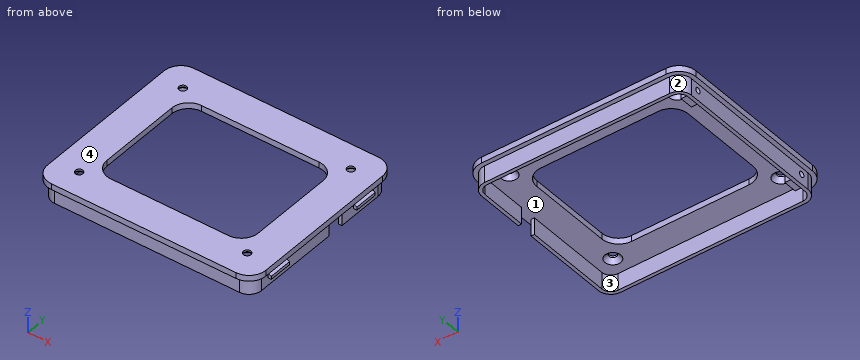
from build123d import *

# Parameters (mm, degrees)
P_IDAT_VYSUNUT_M2_DEPTH                           = 3.5
P_IDAT_VYSUNUT_M3_DEPTH                           = 10
V_LCOV_ZAHLOUBEN_PRO_M4_ROUBY_S_P_2_COUNT         = 2
V_LCOV_ZAHLOUBEN_PRO_M4_ROUBY_S_P_2_PITCH         = 100
V_LCOV_ZAHLOUBEN_PRO_M4_ROUBY_S_P_3_COUNT         = 2
V_LCOV_ZAHLOUBEN_PRO_M4_ROUBY_S_P_3_PITCH         = 128.062484749
V_LCOV_ZAHLOUBEN_PRO_M4_ROUBY_S_P_4_COUNT         = 2
V_LCOV_ZAHLOUBEN_PRO_M4_ROUBY_S_P_4_PITCH         = 80
ODEBRAT_VYSUNUT_M2_DEPTH                          = 86.732140997
SKICA8_W                                          = 5
SKICA8_H                                          = 8
SKICA8_W_2                                        = 3
SKICA8_W_3                                        = 8
P_IDAT_VYSUNUT_M4_DEPTH                           = 5
V_LCOV_ZAHLOUBEN_PRO_M3_ROUBY_S_V_LCO_D           = 3.4
V_LCOV_ZAHLOUBEN_PRO_M3_ROUBY_S_V_LCO_DEPTH       = 9.6
V_LCOV_ZAHLOUBEN_PRO_M3_ROUBY_S_V_LCO_CBORE_D     = 3.9
V_LCOV_ZAHLOUBEN_PRO_M3_ROUBY_S_V_LCO_CBORE_DEPTH = 4
SKICA15_W                                         = 2.8
SKICA15_H                                         = 14
P_IDAT_VYSUNUT_M5_DEPTH                           = 2
ZKOSEN_1_SIZE                                     = 2.144506921
ZKOSEN_1_SIZE_2                                   = 1
ZKOSEN_2_SIZE                                     = 1
ZKOSEN_2_SIZE_2                                   = 2.144506921


with BuildPart() as part:
    # Skica1 → Přidat vysunutím2 (new body)
    with BuildSketch(Plane.XY):
        with BuildLine():
            Line((-55, 55), (55, 55))
            ThreePointArc((55, 55), (62.071067812, 52.071067812), (65, 45))
            Line((65, 45), (65, -45))
            ThreePointArc((65, -45), (62.071067812, -52.071067812), (55, -55))
            Line((55, -55), (-55, -55))
            ThreePointArc((-55, -55), (-62.071067812, -52.071067812), (-65, -45))
            Line((-65, -45), (-65, 45))
            ThreePointArc((-65, 45), (-62.071067812, 52.071067812), (-55, 55))
        make_face()
    extrude(amount=P_IDAT_VYSUNUT_M2_DEPTH)

    # Skica3 → Přidat vysunutím3 (add)
    with BuildSketch(Plane(origin=(0, 0, 0), x_dir=(-1, 0, 0), z_dir=(0, 0, -1))):
        with BuildLine():
            Line((-60.4, 17), (-60.4, 45))
            ThreePointArc((-60.4, 45), (-58.818376618, 48.818376618), (-55, 50.4))
            Line((-55, 50.4), (55, 50.4))
            ThreePointArc((55, 50.4), (58.818376618, 48.818376618), (60.4, 45))
            Line((60.4, 45), (60.4, -45))
            ThreePointArc((60.4, -45), (58.818376618, -48.818376618), (55, -50.4))
            Line((55, -50.4), (-55, -50.4))
            ThreePointArc((-55, -50.4), (-58.818376618, -48.818376618), (-60.4, -45))
            Line((-60.4, -45), (-60.4, 7))
            Line((-60.4, 7), (-62.4, 7))
            Line((-62.4, 7), (-62.4, -45))
            ThreePointArc((-62.4, -45), (-60.232590181, -50.232590181), (-55, -52.4))
            Line((-55, -52.4), (55, -52.4))
            ThreePointArc((55, -52.4), (60.232590181, -50.232590181), (62.4, -45))
            Line((62.4, -45), (62.4, 45))
            ThreePointArc((62.4, 45), (60.232590181, 50.232590181), (55, 52.4))
            Line((55, 52.4), (-55, 52.4))
            ThreePointArc((-55, 52.4), (-60.232590181, 50.232590181), (-62.4, 45))
            Line((-62.4, 45), (-62.4, 17))
            Line((-62.4, 17), (-60.4, 17))
        make_face()
    extrude(amount=P_IDAT_VYSUNUT_M3_DEPTH)

    # Skica5 → Válcové zahloubení pro M4 šrouby s plochou hlavou1 (revolve, cut)
    with BuildSketch(Plane(origin=(-50, -40, 0), x_dir=(0, 1, 0), z_dir=(1, 0, 0))):
        Polygon((0, 0), (0, 3.5), (2.25, 3.5), (2.25, 2.45), (4.7, 0), align=None)
    v_lcov_zahlouben_pro_m4_rouby_s_ploch = revolve(axis=Axis((-50, -40, -6.35), (0, 0, 1)), mode=Mode.SUBTRACT)

    # V_lcov_ zahlouben_ pro M4 _rouby s p 2: Válcové zahloubení pro M4 šrouby s plochou hlavou1 ×2
    with Locations(*[(i * V_LCOV_ZAHLOUBEN_PRO_M4_ROUBY_S_P_2_PITCH, 0, 0) for i in range(1, V_LCOV_ZAHLOUBEN_PRO_M4_ROUBY_S_P_2_COUNT)]):
        add(v_lcov_zahlouben_pro_m4_rouby_s_ploch, mode=Mode.SUBTRACT)

    # V_lcov_ zahlouben_ pro M4 _rouby s p 3: Válcové zahloubení pro M4 šrouby s plochou hlavou1 ×2
    with Locations(*[Vector(0.7808688094430304, 0.6246950475544243, 0) * (i * V_LCOV_ZAHLOUBEN_PRO_M4_ROUBY_S_P_3_PITCH) for i in range(1, V_LCOV_ZAHLOUBEN_PRO_M4_ROUBY_S_P_3_COUNT)]):
        add(v_lcov_zahlouben_pro_m4_rouby_s_ploch, mode=Mode.SUBTRACT)

    # V_lcov_ zahlouben_ pro M4 _rouby s p 4: Válcové zahloubení pro M4 šrouby s plochou hlavou1 ×2
    with Locations(*[(0, i * V_LCOV_ZAHLOUBEN_PRO_M4_ROUBY_S_P_4_PITCH, 0) for i in range(1, V_LCOV_ZAHLOUBEN_PRO_M4_ROUBY_S_P_4_COUNT)]):
        add(v_lcov_zahlouben_pro_m4_rouby_s_ploch, mode=Mode.SUBTRACT)

    # Skica6 → Odebrat vysunutím2 (cut, through all)
    with BuildSketch(Plane(origin=(0, 0, 0), x_dir=(-1, 0, 0), z_dir=(0, 0, -1))):
        with BuildLine():
            Line((-35, -35), (35, -35))
            ThreePointArc((35, -35), (42.071067812, -32.071067812), (45, -25))
            Line((45, -25), (45, 25))
            ThreePointArc((45, 25), (42.071067812, 32.071067812), (35, 35))
            Line((35, 35), (-35, 35))
            ThreePointArc((-35, 35), (-42.071067812, 32.071067812), (-45, 25))
            Line((-45, 25), (-45, -25))
            ThreePointArc((-45, -25), (-42.071067812, -32.071067812), (-35, -35))
        make_face()
    extrude(amount=-ODEBRAT_VYSUNUT_M2_DEPTH, mode=Mode.SUBTRACT)

    # Skica8 → Přidat vysunutím4 (add)
    with BuildSketch(Plane(origin=(-60.4, 0, 0), x_dir=(0, 0, -1), z_dir=(1, 0, 0))):
        with Locations((2.5, 40)):
            Rectangle(SKICA8_W, SKICA8_H)
        with Locations((6.5, 40)):
            Rectangle(SKICA8_W_2, SKICA8_H)
        with Locations((4, -40)):
            Rectangle(SKICA8_W_3, SKICA8_H)
    extrude(amount=P_IDAT_VYSUNUT_M4_DEPTH)

    # Válcové zahloubení pro M3 šrouby s válcovou hlavou zaoblenou1
    with Locations(Plane(origin=(-55.4, 40, -4), x_dir=(0, 0, 1), z_dir=(1, 0, 0))):
        with Locations((0, 0)):
            v_lcov_zahlouben_pro_m3_rouby_s_v_lco = CounterBoreHole(V_LCOV_ZAHLOUBEN_PRO_M3_ROUBY_S_V_LCO_D / 2, V_LCOV_ZAHLOUBEN_PRO_M3_ROUBY_S_V_LCO_CBORE_D / 2, V_LCOV_ZAHLOUBEN_PRO_M3_ROUBY_S_V_LCO_CBORE_DEPTH, depth=V_LCOV_ZAHLOUBEN_PRO_M3_ROUBY_S_V_LCO_DEPTH)

    # Zrcadlit1: Válcové zahloubení pro M3 šrouby s válcovou hlavou zaoblenou1 across plane
    add(v_lcov_zahlouben_pro_m3_rouby_s_v_lco.mirror(Plane.ZX), mode=Mode.SUBTRACT)

    # Skica15 → Přidat vysunutím5 (add)
    with BuildSketch(Plane(origin=(62.4, 0, 0), x_dir=(0, 0, -1), z_dir=(1, 0, 0))):
        with Locations((4, 33)):
            Rectangle(SKICA15_W, SKICA15_H)
        with Locations((4, -33)):
            Rectangle(SKICA15_W, SKICA15_H)
    extrude(amount=P_IDAT_VYSUNUT_M5_DEPTH)

    # Zkosení1
    # the kernel refuses this chamfer: 2.144506921, 1 mm, written as the material it takes off along each edge
    with BuildSketch(Plane(origin=(64.4, -45.556364829, -2.6), x_dir=(-0.9998669641130703, 0, 0.016311164131110292), z_dir=(0, 1, 0))) as zkosen_1_piece_1_section:
        Polygon((ZKOSEN_1_SIZE * 0.999866963884, -ZKOSEN_1_SIZE * 0.0163111641274), (-ZKOSEN_1_SIZE_2 * 0.0163111641311, -ZKOSEN_1_SIZE_2 * 0.999866964113), (0, 0), align=None)
    zkosen_1_piece_1 = extrude(amount=25.112729659, mode=Mode.PRIVATE)
    zkosen_1_piece_1 = split(zkosen_1_piece_1, bisect_by=Plane(origin=(62.4, -33, -2.920893851), z_dir=(1, 0, 0)), keep=Keep.TOP, mode=Mode.PRIVATE)
    add(zkosen_1_piece_1, mode=Mode.SUBTRACT)

    # Zkosení2
    # the kernel refuses this chamfer: 2.144506921, 1 mm, written as the material it takes off along each edge
    with BuildSketch(Plane(origin=(64.4, 20.443635171, -2.6), x_dir=(0.07481330637059905, 0, -0.9971975577536776), z_dir=(0, 1, 0))) as zkosen_2_piece_1_section:
        Polygon((ZKOSEN_2_SIZE * 0.997197557754, ZKOSEN_2_SIZE * 0.0748133063706), (-ZKOSEN_2_SIZE_2 * 0.0748133063535, ZKOSEN_2_SIZE_2 * 0.997197557526), (0, 0), align=None)
    zkosen_2_piece_1 = extrude(amount=25.112729659, mode=Mode.PRIVATE)
    zkosen_2_piece_1 = split(zkosen_2_piece_1, bisect_by=Plane(origin=(62.4, 33, -2.920893851), z_dir=(1, 0, 0)), keep=Keep.TOP, mode=Mode.PRIVATE)
    add(zkosen_2_piece_1, mode=Mode.SUBTRACT)


solid = part.part
The listing builds one solid part. Answer for the finished solid, in the listing's coordinates (mm). Face numbers are marked on the shaded views. Round coordinates to 2 decimals unless told otherwise and drop trailing zeros. Write each loop counter-clockwise with the first axis right and the second up, starting at its lowest first coordinate (ties: lowest second). Pieces come first, ordered by that corner, then holes. Notation, with made-up numbers: M 47,78 L 51,78 A22 cw 51,108 Z; hole C 26.25,-34 d5. An arc over 180 degrees is marked long. Write each question's results on one line, items separated by ' | '. Start each with the question number.
Item 1: Flat-ended cylindrical pins translate along their axes: pin 1 Ø4 at (y, z) = (40, -4) entering from +X; pin 2 Ø2 at (x, z) = (62, -6) entering from -Y; pin 3 Ø2 at (x, z) = (63.5, -3.5) entering from -Y; pin 4 Ø4 at (x, y) = (-50, 40) entering from -Z. Find the tip coordinate at first contact, or state that the pin passes through.
Item 2: A cutting plane is placed at A-A on y = 9. Write down the section's boundary in (x, z).
Item 3: For a pull along X with two mould halves and no side action, classify the marked faces 1, 2, 3 and 4 as pulls with the +X half, pulls with the -X half, needs draft (parallel to the pull), parting line crosses it, or undercut.
Item 4: Straight lines are drawn through the part: L1, parallel to Y at x = -50, z = 2.95; L2, parallel to X at y = -21.5, z = 0.25; L3, parallel to Y at x = 10, z = -6.5. For each, find the intervals that lie inside material, in ascending order. Write a range as [from, to].
Item 5: A cutting plane is placed at D-D on y = 22.5. Write down the section's boundary in (x, z), and give its area (3 significant figures).
Item 6: A cutting plane is placed at C-C on x = -50. Write down the section's boundary in (y, z), and give its area (3 significant figures).
Item 7: A cutting plane is placed at B-B on x = -11. Write down the section's boundary in (y, z).
Check sheet entries:
1) pin 1: x = 64.4 | pin 2: y = -49.33 | pin 3: y = -40 | pin 4: through
2) outline: M -65,0 L -62.4,0 L -62.4,-10 L -60.4,-10 L -60.4,0 L -45,0 L -45,3.5 L -65,3.5 Z; M 45,0 L 65,0 L 65,3.5 L 45,3.5 Z
3) face 1: undercut | face 2: pulls with the -X half | face 3: undercut | face 4: needs draft
4) L1: [-55, -42.25], [-37.75, 37.75], [42.25, 55] | L2: [-65, -45], [45, 65] | L3: [-52.4, -50.4], [50.4, 52.4]
5) outline: M -65,0 L -62.4,0 L -62.4,-10 L -60.4,-10 L -60.4,0 L -45,0 L -45,3.5 L -65,3.5 Z; M 45,0 L 60.4,0 L 60.4,-10 L 62.4,-10 L 62.4,0 L 65,0 L 65,3.5 L 45,3.5 Z | area: 180 mm²
6) outline: M -55,0 L -52.4,0 L -52.4,-10 L -50.4,-10 L -50.4,0 L -44.7,0 L -42.25,2.45 L -42.25,3.5 L -55,3.5 Z; M -37.75,2.45 L -35.3,0 L 35.3,0 L 37.75,2.45 L 37.75,3.5 L -37.75,3.5 Z; M 42.25,2.45 L 44.7,0 L 50.4,0 L 50.4,-10 L 52.4,-10 L 52.4,0 L 55,0 L 55,3.5 L 42.25,3.5 Z | area: 381 mm²
7) outline: M -55,0 L -52.4,0 L -52.4,-10 L -50.4,-10 L -50.4,0 L -35,0 L -35,3.5 L -55,3.5 Z; M 35,0 L 50.4,0 L 50.4,-10 L 52.4,-10 L 52.4,0 L 55,0 L 55,3.5 L 35,3.5 Z
